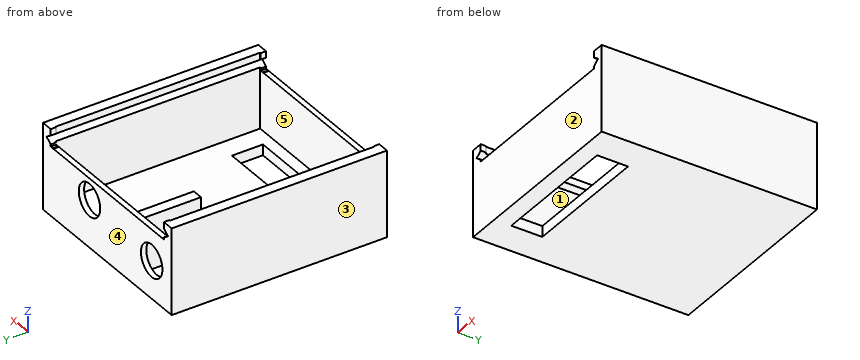
```python
from build123d import *

# Parameters (mm, degrees)
F0_W      = 45.72
F0_H      = 50.8
F1_DEPTH  = 20.32
F2_W      = 40.64
F2_H      = 48.26
F3_DEPTH  = 17.78
F6_DEPTH  = 76.2
F7_W      = 40.2336
F7_H      = 13.4213150721
F8_DEPTH  = 76.2
F9_R      = 3.81
F10_DEPTH = 25.4
F11_R     = 3.81
F12_DEPTH = 25.4
F13_W     = 30.48
F13_H     = 7.3176570747
F14_DEPTH = 25.4
F16_W     = 85.4751653969
F16_H     = 36.5072973073
F17_DEPTH = 27.4827411682
F4_W      = 45.72
F4_H      = 20.32
F18_DEPTH = 1295.4
F19_W     = 2.54
F19_H     = 14.0831380416
F20_DEPTH = 12.7


with BuildPart() as f1:
    # F0 (on Top) → F1 (new body)
    with BuildSketch(Plane.XY):
        with Locations((0.3116804636, 2.0817411682)):
            Rectangle(F0_W, F0_H)
    extrude(amount=F1_DEPTH)

    # F2 (on face) → F3 (cut)
    with BuildSketch(Plane(origin=(0, 0, 0), x_dir=(1, 0, 0), z_dir=(0, 0, -1))):
        with Locations((0.3116804636, -2.0817411682)):
            Rectangle(F2_W, F2_H)
    extrude(amount=-F3_DEPTH, mode=Mode.SUBTRACT)

    # F5 (on face) → F6 (cut)
    with BuildSketch(Plane(origin=(0, 27.4817411682, 0), x_dir=(-1, 0, 0), z_dir=(0, 1, 0))):
        Polygon((7.4571696945, -7.1376733061), (21.2783195364, 2.54), (19.0544535564, 4.0971677232), align=None)
        Polygon((-16.4789422694, -1.2570421612), (-19.511084422, 4.2139133691), (-21.9016804636, 2.54), align=None)
    extrude(amount=-F6_DEPTH, mode=Mode.SUBTRACT)

    # F7 (on face) → F8 (cut)
    with BuildSketch(Plane(origin=(0, 27.4817411682, 0), x_dir=(-1, 0, 0), z_dir=(0, 1, 0))):
        with Locations((-0.3116804636, -2.6208243798)):
            Rectangle(F7_W, F7_H)
    extrude(amount=-F8_DEPTH, mode=Mode.SUBTRACT)

    # F9 (on face) → F10 (cut)
    with BuildSketch(Plane(origin=(0, 27.4817411682, 0), x_dir=(-1, 0, 0), z_dir=(0, 1, 0))):
        with Locations((-6.658220198, 9.1409003362)):
            Circle(F9_R)
    extrude(amount=-F10_DEPTH, mode=Mode.SUBTRACT)

    # F11 (on face) → F12 (cut)
    with BuildSketch(Plane(origin=(0, 27.4817411682, 0), x_dir=(-1, 0, 0), z_dir=(0, 1, 0))):
        with Locations((15.4363195364, 11.43)):
            Circle(F11_R)
    extrude(amount=-F12_DEPTH, mode=Mode.SUBTRACT)

    # F13 (on face) → F14 (cut)
    with BuildSketch(Plane.XY.offset(20.32)):
        with Locations((0.3116804636, -15.6860221177)):
            Rectangle(F13_W, F13_H)
    extrude(amount=-F14_DEPTH, mode=Mode.SUBTRACT)

    # F15: F1 across plane


with BuildPart() as f1_1:
    add(f1.part)
    add(f1.part.mirror(Plane.XY))

    # F16 (on Front) → F17 (cut, through all)
    with BuildSketch(Plane.XZ):
        with Locations((-9.5093864948, 18.2536486536)):
            Rectangle(F16_W, F16_H)
    extrude(amount=-F17_DEPTH, mode=Mode.SUBTRACT)

    # F4 (on face) → F18 (cut)
    with BuildSketch(Plane(origin=(0, 27.4817411682, 0), x_dir=(-1, 0, 0), z_dir=(0, 1, 0))):
        with Locations((-0.3116804636, 10.16)):
            Rectangle(F4_W, F4_H)
    extrude(amount=-F18_DEPTH, mode=Mode.SUBTRACT)

    # F19 (on face) → F20 (join)
    with BuildSketch(Plane.XY.offset(-17.78)):
        with Locations((-8.5783195364, 19.1701721474)):
            Rectangle(F19_W, F19_H)
    extrude(amount=F20_DEPTH)


solid = f1_1.part
```
Verification items for the finished model (mm, model axes). Face numbers are marked on the shaded views. A direction names the side the tool comes from. Give positions to 0.01 mm unless a question says otherwise; leave off trailing zeros. Loops run counter-clockwise (first coordinate to the right, second up) from the corner with the lowest first, then second, coordinate; pieces in that order, holes last. Notation, with made-up numbers: M -36.5,65 L -13.5,65 A19 ccw -13.5,90 Z; hole C -19.5,1 d5. An arc over 180 degrees is marked long. One line per question, with ' | ' between items.
Item 1: Thickness scan on line 1 (X direction, y = 14, z = -15.75); line 2 (X direction, y = -20, z = -5.75); line 3 (X direction, y = -19, z = -18.25). Record the ranges inside material, lowest first. Write a range as [from, to].
Completed:
line 1: x = [-22.55, -20.01], [-9.85, -7.31], [20.63, 23.17] | line 2: x = [-22.55, -20.01], [20.63, 23.17] | line 3: x = [-22.55, -14.93], [15.55, 23.17]
Item 2: Section check C-C, the plane y = -17.5. Record the cut outline in (x, z).
Completed:
outline: M -22.55,-20.32 L -14.93,-20.32 L -14.93,-17.78 L -20.01,-17.78 L -20.01,-3.43 L -21.28,-2.54 L -20.01,-1.65 L -20.01,0 L -22.55,0 Z; M 15.55,-20.32 L 23.17,-20.32 L 23.17,0 L 20.63,0 L 20.63,-1.65 L 21.9,-2.54 L 20.63,-3.43 L 20.63,-17.78 L 15.55,-17.78 Z
Item 3: Section check B-B, the plane z = -11.43. Record the cut outline in (x, y), plus the area to 3 significant figures.
Completed:
outline: M -22.55,-23.32 L 23.17,-23.32 L 23.17,27.48 L 9.7,27.48 L 9.7,26.21 L 20.63,26.21 L 20.63,-22.05 L -20.01,-22.05 L -20.01,26.21 L -19.25,26.21 L -19.25,27.48 L -22.55,27.48 Z; M -11.63,26.21 L -9.85,26.21 L -9.85,12.13 L -7.31,12.13 L -7.31,26.21 L 3.61,26.21 L 3.61,27.48 L -11.63,27.48 Z | area: 380 mm^2
Item 4: Depth check by flat-ended pin: P1, Ø3, axis at x = -12, y = -2, coming from the +Z side; P2, Ø1, axis at x = 3.5, y = -17, coming from the -Z side; P3, Ø0.8, axis at x = -19.5, y = -22.5, coming from the +Z side. Enter the tip coordinate at first touch or a pass-through.
Completed:
P1: stops at z = -17.78 | P2: passes through | P3: stops at z = 0
Item 5: Section check A-A, the plane x = -1.5. Record the cut outline in (y, z), plus the area to 3 significant figures.
Completed:
outline: M -23.32,-20.32 L -19.34,-20.32 L -19.34,-17.78 L -22.05,-17.78 L -22.05,-4.09 L -23.32,-4.09 Z; M -12.03,-20.32 L 27.48,-20.32 L 27.48,-4.09 L 26.21,-4.09 L 26.21,-17.78 L -12.03,-17.78 Z | area: 145 mm^2
Item 6: Draft check along X on the marked faces 3, 4 and 5. Enter one of: +X half, -X half, draft (parallel to the pull), parting line (faces both ways), or undercut.
Completed:
face 3: -X half | face 4: draft | face 5: undercut
Item 7: Section check D-D, the plane y = 2. Record the cut outline in (x, z), plus the area to 3 significant figures.
Completed:
outline: M -22.55,-20.32 L 23.17,-20.32 L 23.17,0 L 20.63,0 L 20.63,-1.65 L 21.9,-2.54 L 20.63,-3.43 L 20.63,-17.78 L -20.01,-17.78 L -20.01,-3.43 L -21.28,-2.54 L -20.01,-1.65 L -20.01,0 L -22.55,0 Z | area: 204 mm^2
Item 8: Tool access check on the marked faces 1 and 2. Record the directions out of +Z, -Z, +X, -X, +Y, -Y that give a thin tool (end or side, any length) a straight path to the whole face; none if there is none.
Completed:
face 1: +Z | face 2: +Z, -Z, +X, -X, -Y
